Could you check a few things on this drawing? It's one solid part, dimensions in mm from its lowest x, y, z. A direction names the side the tool comes from. Give positions to 0.01 mm unless a question says otherwise; leave off trailing zeros. Loops run counter-clockwise (first coordinate to the right, second up) from the corner with the lowest first, then second, coordinate; pieces in that order, holes last. Notation, with made-up numbers: (28, 45.25) - (40, 45.25) arc R29 cw to (40, 70.25) - close; hole circle Ø3 at (24.25, 12.5). An arc over 180 degrees is marked (long way). Put each result on its own line as item: value. Start each with the question number.
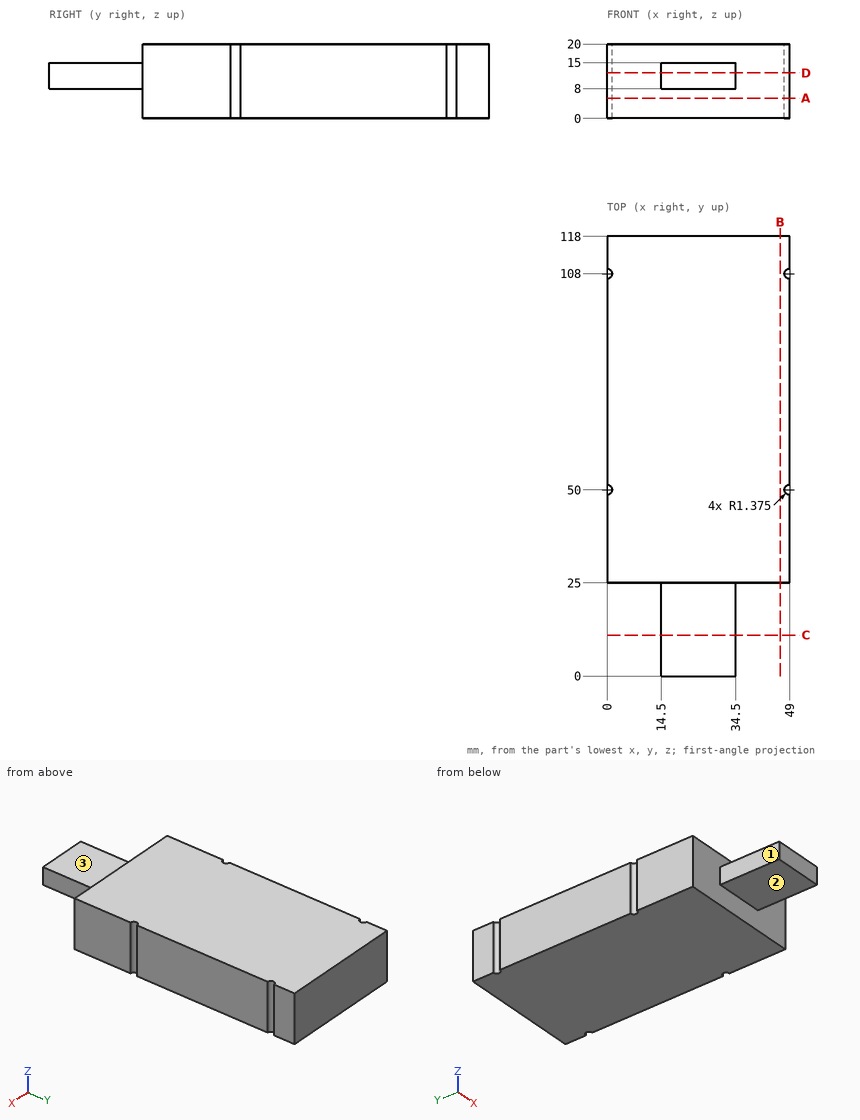
1) Suppose I cut it at A-A on z = 5.5. Please give me the cut outline in (x, y) (3 decimals).
2) Suppose I cut it at D-D on z = 12.25. Please give me the cut outline in (x, y) (3 decimals).
3) I need wall thicknesses on line 1 (X direction, y = 6, z = 8.75); line 2 (Y direction, x = 6, z = 2.25); line 3 (Z direction, x = 31.5, y = 6.5). Which ranges of each line are inside material? Lowest first, please.
4) Which directions (+Z, -Z, +X, -X, +Y, -Y) give clear straight access to the entire face, cutting with the end or side of a thin tool? Please do the marked faces 1, 2 and 3.
5) Suppose I cut it at B-B on x = 46.5. Please give me the cut outline in (y, z).
6) Suppose I cut it at C-C on y = 11. Please give me the cut outline in (x, z), plus the area to 3 significant figures.
7) I'm going to push flat-ended pins straight in: P1, Ø16, axis at x = 26.5, y = 10.5, coming from the +Z side; P2, Ø3.5, axis at y = 13, z = 11.5, coming from the -X side; P3, Ø7.5, axis at y = 13, z = 11.5, coming from the +X side. Where does each tip first touch, or does it pass through?
Ans:
1. outline: (0, 25) - (49, 25) - (49, 48.625) arc R1.375 cw to (49, 51.375) - (49, 106.625) arc R1.375 cw to (49, 109.375) - (49, 118) - (0, 118) - (0, 109.375) arc R1.375 cw to (0, 106.625) - (0, 51.375) arc R1.375 cw to (0, 48.625) - close
2. outline: (0, 25) - (14.5, 25) - (14.5, 0) - (34.5, 0) - (34.5, 25) - (49, 25) - (49, 48.625) arc R1.375 cw to (49, 51.375) - (49, 106.625) arc R1.375 cw to (49, 109.375) - (49, 118) - (0, 118) - (0, 109.375) arc R1.375 cw to (0, 106.625) - (0, 51.375) arc R1.375 cw to (0, 48.625) - close
3. line 1: x = 14.5 to 34.5
3. line 2: y = 25 to 118
3. line 3: z = 8 to 15
4. face 1: +Z, -Z, -X, -Y
4. face 2: -Z, +X, -X, -Y
4. face 3: +Z, +X, -X, -Y
5. outline: (25, 0) - (118, 0) - (118, 20) - (25, 20) - close
6. outline: (14.5, 8) - (34.5, 8) - (34.5, 15) - (14.5, 15) - close
6. area: 140 mm²
7. P1: stops at z = 15
7. P2: stops at x = 14.5
7. P3: stops at x = 34.5
